Part model, mm, in its own coordinate system. A direction names the side the tool comes from. Coordinates: 2 decimals unless noted, no trailing zeros. Order: outer loops, then holes, each group sorted by start corner. A loop starts at its lowest first (then second) coordinate and runs counter-clockwise, first axis right, second up.
```python
from build123d import *

# Parameters (mm, degrees)
SKETCH_1_W          = 50
SKETCH_1_H          = 70
EXTRUDE_1_DEPTH     = 10
SKETCH_2_W          = 10
SKETCH_2_H          = 70
EXTRUDE_2_DEPTH     = 34
SKETCH_3_R          = 11
CUT_EXTRUDE_1_DEPTH = 32
SKETCH_4_R          = 2.25
CUT_EXTRUDE_2_DEPTH = 93.498648639
SKETCH_5_R          = 2.25
CUT_EXTRUDE_3_DEPTH = 93.498648639
SKETCH_6_W          = 34
SKETCH_6_H          = 15
CUT_EXTRUDE_4_DEPTH = 92.847700026
SKETCH_7_W          = 15
SKETCH_7_H          = 15
CUT_EXTRUDE_5_DEPTH = 93.498648639


with BuildPart() as part:
    # 草图1 → 凸台-拉伸1 (new body)
    with BuildSketch(Plane.XY):
        with Locations((25, 35)):
            Rectangle(SKETCH_1_W, SKETCH_1_H)
    extrude(amount=EXTRUDE_1_DEPTH)

    # 草图2 → 凸台-拉伸2 (add)
    with BuildSketch(Plane.XY.offset(10)):
        with Locations((5, 35)):
            Rectangle(SKETCH_2_W, SKETCH_2_H)
    extrude(amount=EXTRUDE_2_DEPTH)

    # 草图3 → 切除-拉伸1 (cut)
    with BuildSketch(Plane(origin=(10, 0, 0), x_dir=(0, 0, -1), z_dir=(1, 0, 0))):
        with Locations(Location((-29, 35, 0), (0, 0, 90))):
            Circle(SKETCH_3_R)
    extrude(amount=-CUT_EXTRUDE_1_DEPTH, mode=Mode.SUBTRACT)

    # 草图4 → 切除-拉伸2 (cut, through all)
    with BuildSketch(Plane.XY.offset(10)):
        with Locations((40, 11.5)):
            Circle(SKETCH_4_R)
        with Locations(Location((40, 58.5, 0), (0, 0, 180))):
            Circle(SKETCH_4_R)
    extrude(amount=-CUT_EXTRUDE_2_DEPTH, mode=Mode.SUBTRACT)

    # 草图5 → 切除-拉伸3 (cut, through all)
    with BuildSketch(Plane.XY.offset(10)):
        with Locations((35, 66)):
            Circle(SKETCH_5_R)
        with Locations(Location((35, 4, 0), (0, 0, 180))):
            Circle(SKETCH_5_R)
        with Locations((29, 4)):
            Circle(SKETCH_5_R)
        with Locations(Location((29, 66, 0), (0, 0, 180))):
            Circle(SKETCH_5_R)
    extrude(amount=-CUT_EXTRUDE_3_DEPTH, mode=Mode.SUBTRACT)

    # 草图6 → 切除-拉伸4 (cut, through all)
    with BuildSketch(Plane(origin=(10, 0, 0), x_dir=(0, 0, -1), z_dir=(1, 0, 0))):
        with Locations((-27, 7.5)):
            Rectangle(SKETCH_6_W, SKETCH_6_H)
        with Locations((-27, 62.5)):
            Rectangle(SKETCH_6_W, SKETCH_6_H)
    extrude(amount=-CUT_EXTRUDE_4_DEPTH, mode=Mode.SUBTRACT)

    # 草图7 → 切除-拉伸5 (cut, through all)
    with BuildSketch(Plane.XY.offset(10)):
        with Locations((7.5, 7.5)):
            Rectangle(SKETCH_7_W, SKETCH_7_H)
        with Locations((7.5, 62.5)):
            Rectangle(SKETCH_7_W, SKETCH_7_H)
    extrude(amount=-CUT_EXTRUDE_5_DEPTH, mode=Mode.SUBTRACT)


solid = part.part
```
(1) Slice it at C-C, the plane z = 29. Give the cut face in (x, y), then the cut area to 3 significant figures.
(2) Slice it at D-D, the plane y = 4. Give the cut face in (x, z).
(3) Tool access for faces 4 (the face through (30, 35, 10)), 5 (the face through (6, 55, 22)), 6 (the face through (6, 15, 22)), 7 (the face through (5, 35, 44)): list every direction of +Z, -Z, +X, -X, +Y, -Y with a clear straight run to the whole face (end or side of a thin tool).
(4) Pull direction Z, two halves, no side cores. Call faces 1 (the face through (5.07, 26.27, 22.31)), 2 (the face through (32, 70, 5)), 3 (the face through (25, 35, 0)): +Z half, -Z half, draft (parallel to the pull), parting line (faces both ways), or undercut.
(5) Slice it at A-A, the plane x = 40. Give the cut face in (y, z), then the cut area to 3 significant figures.
(6) Slice it at B-B, the plane y = 11.5. Give the cut face in (x, z).
(7) Drop flat-ended pins along their axis: pin 1 (7.5 mm diameter, centred on x = 8.5, z = 20, fed in from +Y); pin 2 (5 mm diameter, centred on y = 26, z = 35.5, fed in from -X); pin 3 (20 mm diameter, centred on x = 20.5, y = 50.5, fed in from +Z); pin 4 (12 mm diameter, centred on y = 18.5, z = 31.5, fed in from +X). Give the stop position or say it passes through.
(8) Probe line 1 (Y direction, x = 40, z = 2.75); line 2 (Y direction, x = 35, z = 6); line 3 (Z direction, x = 4, y = 35). List the from-to ranges inside material, lowest first.
Here are the results:
1. outline: (0, 15) - (10, 15) - (10, 24) - (0, 24) - close; (0, 46) - (10, 46) - (10, 55) - (0, 55) - close
1. area: 180 mm2
2. outline: (15, 0) - (26.75, 0) - (26.75, 10) - (15, 10) - close; (31.25, 0) - (32.75, 0) - (32.75, 10) - (31.25, 10) - close; (37.25, 0) - (50, 0) - (50, 10) - (37.25, 10) - close
3. face 4: +Z, +X, +Y, -Y
3. face 5: +Z, -Z, -X, +Y
3. face 6: +Z, -Z, -X, -Y
3. face 7: +Z, +X, -X, +Y, -Y
4. face 1: undercut
4. face 2: draft
4. face 3: -Z half
5. outline: (0, 0) - (9.25, 0) - (9.25, 10) - (0, 10) - close; (13.75, 0) - (56.25, 0) - (56.25, 10) - (13.75, 10) - close; (60.75, 0) - (70, 0) - (70, 10) - (60.75, 10) - close
5. area: 610 mm2
6. outline: (15, 0) - (37.75, 0) - (37.75, 10) - (15, 10) - close; (42.25, 0) - (50, 0) - (50, 10) - (42.25, 10) - close
7. pin 1: stops at y = 55
7. pin 2: stops at x = 0
7. pin 3: stops at z = 10
7. pin 4: stops at x = 10
8. line 1: y = 0 to 9.25, 13.75 to 56.25, 60.75 to 70
8. line 2: y = 0 to 1.75, 6.25 to 63.75, 68.25 to 70
8. line 3: z = 0 to 18, 40 to 44
